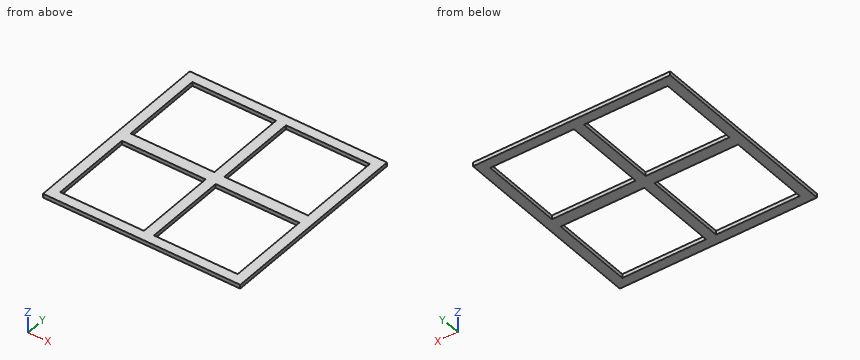
```python
from build123d import *

# Parameters (mm, degrees)
F0_W     = 100
F0_H     = 100
F0_W_2   = 42.465364635
F0_H_2   = 5.9141498059
F0_W_3   = 5.06927073
F0_H_3   = 42.042925097
F1_DEPTH = 2


with BuildPart() as f1:
    # F0 (on Top) → F1 (new body)
    with BuildSketch(Plane.XY):
        Rectangle(F0_W, F0_H)
        Polygon((2.534635365, 45), (45, 45), (45, 2.957074903), (45, -2.957074903), (45, -45), (2.534635365, -45), (-2.534635365, -45), (-45, -45), (-45, -2.957074903), (-45, 2.957074903), (-45, 45), (-2.534635365, 45), align=None, mode=Mode.SUBTRACT)
        with Locations((-23.7673176825, 0)):
            Rectangle(F0_W_2, F0_H_2)
        with Locations((23.7673176825, 0)):
            Rectangle(F0_W_2, F0_H_2)
        with Locations((0, 23.9785374515)):
            Rectangle(F0_W_3, F0_H_3)
        with Locations((0, -23.9785374515)):
            Rectangle(F0_W_3, F0_H_3)
        Rectangle(F0_W_3, F0_H_2)
    extrude(amount=F1_DEPTH)


solid = f1.part
```
CAD build for the part. Positions are in the model's coordinates, mm. Round coordinates to 2 decimals unless told otherwise and drop trailing zeros. Loops run counter-clockwise (first coordinate to the right, second up) from the corner with the lowest first, then second, coordinate; pieces in that order, holes last. Notation, with made-up numbers: M -28.75,34.25 L -8.75,34.25 A21 cw -8.75,58.25 Z; hole C 89.25,89 d4. An arc over 180 degrees is marked long. Use a Markdown table: item, result. Add a question column.
(1) Cut at B-B (y = -10.5). Give the cut face in (x, z), and give its area (3 significant figures).
(2) Drill centre lines: line 1 (Y direction, x = 39.5, z = 1.75); line 2 (X direction, y = 38.5, z = 0.9). Where is each one in solid material? Low to high.
(3) Cut at C-C (z = 0.4). Give the cut face in (x, y).
(4) Flat gauge pin, fed straight in: pin 1 (1.5 mm diameter, centred on x = 31, y = -5.5, fed in from -Z). Where does the tip first touch, or does it go through?
(5) Cut at A-A (x = 31). Give the cut face in (y, z), and give its area (3 significant figures).
Geometry says:
| question | item | result |
|---|---|---|
| 1 | outline | M -50,0 L -45,0 L -45,2 L -50,2 Z; M -2.53,0 L 2.53,0 L 2.53,2 L -2.53,2 Z; M 45,0 L 50,0 L 50,2 L 45,2 Z |
| 1 | area | 30.1 mm² |
| 2 | line 1 | y = -50 to -45, -2.96 to 2.96, 45 to 50 |
| 2 | line 2 | x = -50 to -45, -2.53 to 2.53, 45 to 50 |
| 3 | outline | M -50,-50 L 50,-50 L 50,50 L -50,50 Z; hole M -45,-45 L -2.53,-45 L -2.53,-2.96 L -45,-2.96 Z; hole M -45,2.96 L -2.53,2.96 L -2.53,45 L -45,45 Z; hole M 2.53,-45 L 45,-45 L 45,-2.96 L 2.53,-2.96 Z; hole M 2.53,2.96 L 45,2.96 L 45,45 L 2.53,45 Z |
| 4 | pin 1 | passes through |
| 5 | outline | M -50,0 L -45,0 L -45,2 L -50,2 Z; M -2.96,0 L 2.96,0 L 2.96,2 L -2.96,2 Z; M 45,0 L 50,0 L 50,2 L 45,2 Z |
| 5 | area | 31.8 mm² |
